Source: three-view drawing plus pictorial views. Frame: mm from the lowest corner of the part. A direction names the side the tool comes from. Coordinates: 2 decimals unless noted, no trailing zeros. Write each loop counter-clockwise with the first axis right and the second up, starting at its lowest first coordinate (ties: lowest second). Pieces come first, ordered by that corner, then holes. Notation, with made-up numbers: M 84.5,43.5 L 120.5,43.5 A26 cw 120.5,62.5 Z; hole C 78,28.25 d1. An arc over 180 degrees is marked long. Answer as a JSON object with one key per item and string values. Group by question number.
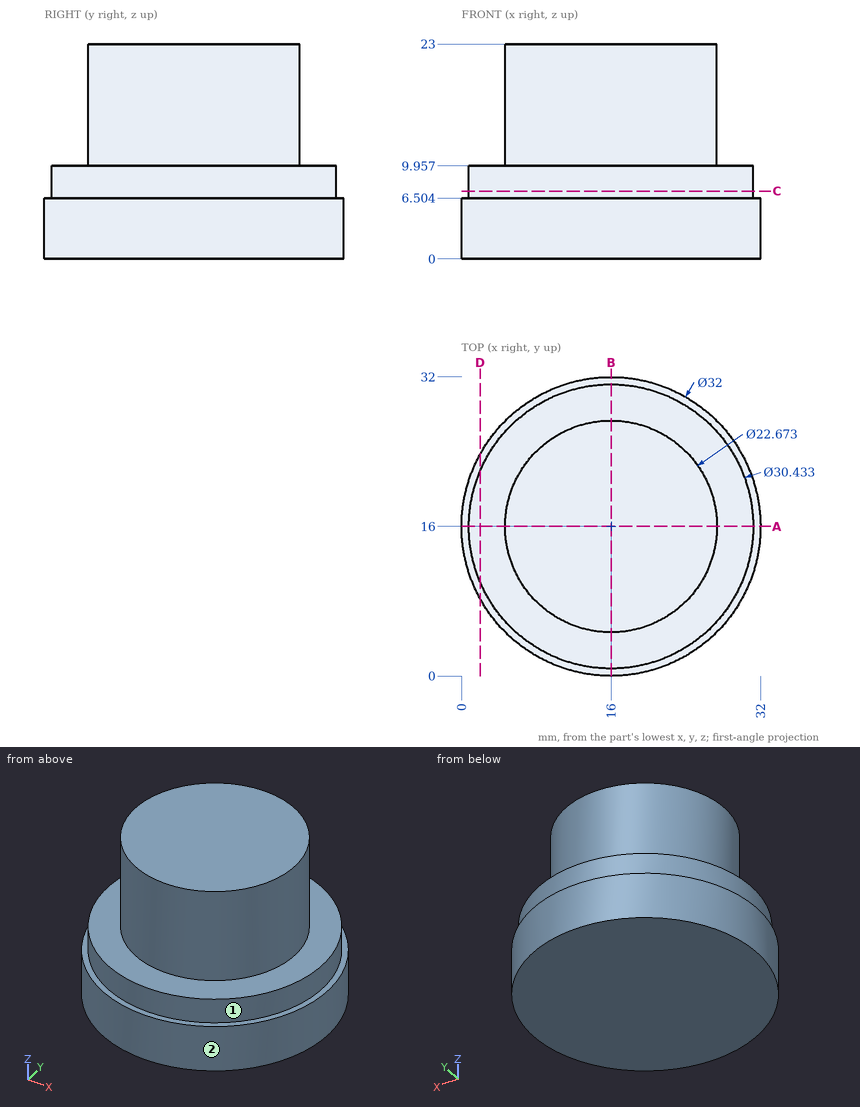
Q1. Section A-A, the plane y = 16. Return the cut outline in (x, z).
Q2. Section D-D, the plane x = 2. Return the cut outline in (y, z).
Q3. Access query for the marked faces 1 and 2. Directions: +Z, -Z, +X, -X, +Y, -Y. A direction counts if a zero-diameter tool reaches every point of the face in a straight line with its end or side. Return the directions, or none.
Q4. Section C-C, the plane z = 7.25. Return the cut outline in (x, y).
Q5. Line query: line 1 (Z direction, x = 24, y = 27); line 2 (Y direction, x = 16.5, z = 8.5); line 3 (X direction, y = 23, z = 14.5). Output: solid intervals per line, ascending. Write a range as from..to.
Q6. Pin query (flat end, axial travel): pin 1 Ø6 at (y, z) = (16, 20) entering from +X; pin 2 Ø2 at (x, y) = (26.5, 8.5) entering from -Z; pin 3 Ø2 at (y, z) = (10, 3) entering from +X; pin 4 Ø10 at (y, z) = (4.5, 14.5) entering from +X (1 decimal). Return the tip coordinate at first contact, or that it passes through.
Filled in:
{
 "1": {"outline": "M 0,0 L 32,0 L 32,6.5 L 31.22,6.5 L 31.22,9.96 L 27.34,9.96 L 27.34,23 L 4.66,23 L 4.66,9.96 L 0.78,9.96 L 0.78,6.5 L 0,6.5 Z"},
 "2": {"outline": "M 8.25,0 L 23.75,0 L 23.75,6.5 L 21.96,6.5 L 21.96,9.96 L 10.04,9.96 L 10.04,6.5 L 8.25,6.5 Z"},
 "3": {"face 1": "+Z", "face 2": "+Z, -Z"},
 "4": {"outline": "C 16,16 d30.43"},
 "5": {"line 1": "0..9.96", "line 2": "0.79..31.21", "line 3": "7.08..24.92"},
 "6": {"pin 1": "x = 27.34", "pin 2": "z = 0", "pin 3": "x = 31.2", "pin 4": "x = 28"}
}
